Autodesk Inventor part; units mm, degrees
ref_plane "YZ Plane" through (0, 0, 0) normal (1, 0, 0) x (0, 1, 0)
ref_plane "XZ Plane" through (0, 0, 0) normal (0, 1, 0) x (-1, 0, 0)
ref_plane "XY Plane" through (0, 0, 0) normal (0, 0, 1) x (1, 0, 0)
sketch "Sketch1" plane through (0, 0, 0) normal (0, 0, 1) x (1, 0, 0)
  circle A0 centre (0, 0) radius 18.1229
  circle A1 centre (0, 0) radius 18.9615
  dimension "d0" = 36.2458
extrude "Extrusion3" add sketch "Sketch1" along normal blind 4.826 contours A0
sketch "Sketch4" plane through (0, 0, 4.826) normal (0, 0, 1) x (1, 0, 0)
  circle A0 centre (0, 0) radius 19.05
  dimension "d17" = 38.1
extrude "Extrusion4" add sketch "Sketch4" along normal blind 1.27
sketch "Sketch5" plane through (0, 0, 0) normal (0, 0, -1) x (-1, 0, 0)
  circle A0 centre (0, 0) radius 19.05
  dimension "d18" = 38.1
extrude "Extrusion5" add sketch "Sketch5" along normal blind 1.27
sketch "Sketch6" plane through (0, 0, 6.096) normal (0, 0, 1) x (1, 0, 0)
  line L0 (2.8729, -2.3622) -> (-2.8729, -2.3622)
  line L1 (2.8729, 2.3622) -> (-2.8729, 2.3622)
  arc A0 (2.8729, -2.3622) -> (2.8729, 2.3622) centre (-1.1303, 0) ccw
  arc A1 (-2.8729, 2.3622) -> (-2.8729, -2.3622) centre (1.1303, 0) ccw
  line L2 (3.5179, 0) -> (-3.5179, 0)
  line L3 (0, 2.3622) -> (0, -2.3622)
  dimension "d23" = 4.7244
  dimension "d24" = 4.6482
  dimension "d25" = 4.6482
  dimension "d26" = 7.0358
extrude "Extrusion7" cut sketch "Sketch6" against normal blind 25.4
properties part number "big tire sumo robot"
Work out the finished part from the listing and answer in its coordinate system (mm). A direction names the side the tool comes from. Give positions to 0.01 mm unless a question says otherwise; leave off trailing zeros. Order: outer loops, then holes, each group sorted by start corner. A loop starts at its lowest first (then second) coordinate and runs counter-clockwise, first axis right, second up. Notation, with made-up numbers: (70.25, 13.5) - (97.25, 13.5) arc R13 ccw to (97.25, 37.5) - close; hole circle Ø7 at (18.25, -32). An arc over 180 degrees is marked (long way). Answer as CSV lines item,"result". Start each with the question number.
Q1. The mould has two halves that part along Z. Classify faces 4 (the face through (-17, -7, 0)), 5 (the face through (15.12, 11.59, -0.63)), 6 (the face through (-4, 0, -1.27)), 7 (the face through (17, -7, 4.826)): +Z half, -Z half, draft (parallel to the pull), parting line (faces both ways), or undercut.
Q2. Find the intervals of material crossed by L1, parallel to Y at x = 0, z = 0.25; L2, parallel to Y at x = -2.5, z = 0.75; L3, parallel to X at y = -12.5, z = 0.75, in increasing order. Write a range as [from, to].
Q3. The part is cut by section C-C (z = 1.25). Write down the section's boundary in (x, y).
Q4. The part is cut by section A-A (x = 0). Write down the section's boundary in (y, z).
Q5. For faces 1 (the face through (-3.9, 17.7, 2.4)), 2 (the face through (-3.518, 0.035, 2.465)), 3 (the face through (4, 0, 6.096)), determine the directions among +Z, -Z, +X, -X, +Y, -Y from which every point of the face is accessible in a straight line to the end or side of a thin tool.
Q6. The part is cut by section B-B (y = 0.5). Write down the section's boundary in (x, z).
Q7. Given pin 1 Ø3 at (y, z) = (-5.5, 1) entering from -X; pin 2 Ø2 at (y, z) = (3.5, 4.5) entering from -X; pin 3 Ø3 at (x, z) = (0.5, 2.5) entering from +Y, each flat-ended and moving along its own axis, determine where each tip first touches the part or whether it passes through.
Q8. The part is cut by section D-D (y = -10). Write down the section's boundary in (x, z).
Check result:
1,face 4,"undercut"
1,face 5,"draft"
1,face 6,"-Z half"
1,face 7,"undercut"
2,L1,"y = [-18.12, -2.36], [2.36, 18.12]"
2,L2,"y = [-17.95, -2.36], [2.36, 17.95]"
2,L3,"x = [-13.12, 13.12]"
3,outline,"circle Ø36.25 at (0, 0); hole (-2.87, -2.36) - (2.87, -2.36) arc R4.65 ccw to (2.87, 2.36) - (-2.87, 2.36) arc R4.65 ccw to start"
4,outline,"(-19.05, -1.27) - (-2.36, -1.27) - (-2.36, 6.1) - (-19.05, 6.1) - (-19.05, 4.83) - (-18.12, 4.83) - (-18.12, 0) - (-19.05, 0) - close; (2.36, -1.27) - (19.05, -1.27) - (19.05, 0) - (18.12, 0) - (18.12, 4.83) - (19.05, 4.83) - (19.05, 6.1) - (2.36, 6.1) - close"
5,face 1,"none"
5,face 2,"+Z, -Z"
5,face 3,"+Z, +X, -X, +Y, -Y"
6,outline,"(-19.04, -1.27) - (-3.49, -1.27) - (-3.49, 6.1) - (-19.04, 6.1) - (-19.04, 4.83) - (-18.12, 4.83) - (-18.12, 0) - (-19.04, 0) - close; (3.49, -1.27) - (19.04, -1.27) - (19.04, 0) - (18.12, 0) - (18.12, 4.83) - (19.04, 4.83) - (19.04, 6.1) - (3.49, 6.1) - close"
7,pin 1,"stops at x = -18.54"
7,pin 2,"stops at x = -18.88"
7,pin 3,"stops at y = 18.12"
8,outline,"(-16.21, -1.27) - (16.21, -1.27) - (16.21, 0) - (15.11, 0) - (15.11, 4.83) - (16.21, 4.83) - (16.21, 6.1) - (-16.21, 6.1) - (-16.21, 4.83) - (-15.11, 4.83) - (-15.11, 0) - (-16.21, 0) - close"
